Geometry: final body of the model. Coordinates: model frame, mm. Round coordinates to 2 decimals unless told otherwise and drop trailing zeros. Loops run counter-clockwise (first coordinate to the right, second up) from the corner with the lowest first, then second, coordinate; pieces in that order, holes last. Notation, with made-up numbers: M 39,19 L 91,19 A27 cw 91,44 Z; hole C -14,49 d9. An arc over 180 degrees is marked long. Answer as a JSON object with one key per item and string values.
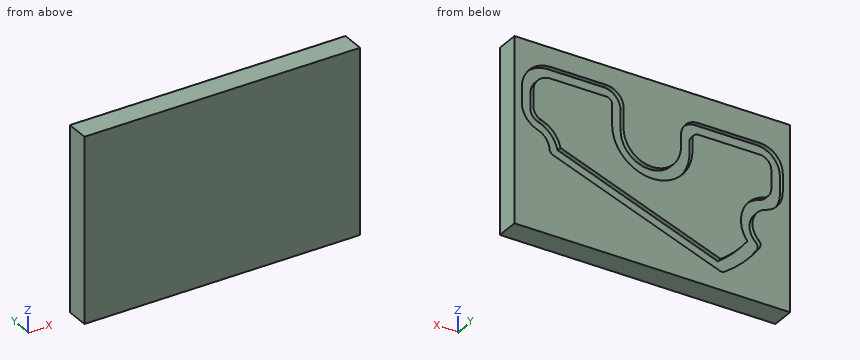
```python
from build123d import *

# Parameters (mm, degrees)
BOSS_EXTRUDE1_DEPTH = 2.54
BOSS_EXTRUDE2_DEPTH = 10.16
BOSS_EXTRUDE4_DEPTH = 2.54
FILLET1_R           = 3.175
FILLET2_R           = 3.175
FILLET3_R           = 3.175


with BuildPart() as part:
    # Sketch1 → Boss-Extrude1 (new body)
    with BuildSketch(Plane(origin=(0, 0, 0), x_dir=(1, 0, 0), z_dir=(0, 1, 0))):
        with BuildLine():
            Line((-59.436, -9.652), (-25.4, -9.652))
            ThreePointArc((-25.4, -9.652), (-23.15493597, -8.72206403), (-22.225, -6.477))
            Line((-22.225, -6.477), (-22.225, 0))
            ThreePointArc((-22.225, 0), (0, 22.225), (22.225, 0))
            Line((22.225, 0), (22.225, -11.049))
            ThreePointArc((22.225, -11.049), (23.15493597, -13.29406403), (25.4, -14.224))
            Line((25.4, -14.224), (56.134, -14.224))
            ThreePointArc((56.134, -14.224), (62.958994652, -11.396994652), (65.786, -4.572))
            Line((65.786, -4.572), (65.786, 3.786270628))
            ThreePointArc((65.786, 3.786270628), (64.573284533, 7.518670343), (61.398344054, 9.825451517))
            ThreePointArc((61.398344054, 9.825451517), (54.523861552, 14.288596243), (50.799961303, 21.590016478))
            Line((50.799961303, 21.590016478), (-37.803944764, 53.839200926))
            ThreePointArc((-37.803944764, 53.839200926), (-45.754351941, 47.268774836), (-52.580093852, 39.536458193))
            ThreePointArc((-52.580093852, 39.536458193), (-49.843866059, 24.02540152), (-61.180505495, 13.091032404))
            ThreePointArc((-61.180505495, 13.091032404), (-64.505522161, 10.809293437), (-65.786, 6.98536286))
            Line((-65.786, 6.98536286), (-65.786, -3.302))
            ThreePointArc((-65.786, -3.302), (-63.926128061, -7.792128061), (-59.436, -9.652))
        make_face()
    extrude(amount=BOSS_EXTRUDE1_DEPTH)

    # Sketch2 → Boss-Extrude2 (add)
    with BuildSketch(Plane.XZ):
        Polygon((-76.199999672, 30.988), (-76.199999672, -70.600237501), (76.199999874, -70.612), (76.200000328, 30.988), align=None)
    extrude(amount=BOSS_EXTRUDE2_DEPTH)

    # Sketch9 → Boss-Extrude4 (add)
    with BuildSketch(Plane(origin=(0, 2.54, 0), x_dir=(1, 0, 0), z_dir=(0, 1, 0))):
        Polygon((76.200000328, -30.988), (76.199999874, 70.612), (-76.199999672, 70.600237501), (-76.199999672, -30.988), align=None)
        with BuildLine():
            Line((15.875, 0), (15.875, -11.049))
            ThreePointArc((15.875, -11.049), (18.664807909, -17.784192091), (25.4, -20.574))
            Line((25.4, -20.574), (56.134, -20.574))
            ThreePointArc((56.134, -20.574), (67.449122713, -15.887122713), (72.136, -4.572))
            Line((72.136, -4.572), (72.136, 3.786270628))
            ThreePointArc((72.136, 3.786270628), (69.710569066, 11.251070057), (63.360688108, 15.864632407))
            ThreePointArc((63.360688108, 15.864632407), (58.26569903, 19.828002779), (56.883535343, 26.133305464))
            Line((56.883535343, 26.133305464), (-38.653299329, 60.905869561))
            ThreePointArc((-38.653299329, 60.905869561), (-51.084372013, 50.931222566), (-61.021650194, 38.47025739))
            ThreePointArc((-61.021650194, 38.47025739), (-55.422413128, 28.186543533), (-62.925010989, 19.196701948))
            ThreePointArc((-62.925010989, 19.196701948), (-69.575044323, 14.633224013), (-72.136, 6.98536286))
            Line((-72.136, 6.98536286), (-72.136, -3.302))
            ThreePointArc((-72.136, -3.302), (-68.416256121, -12.282256121), (-59.436, -16.002))
            Line((-59.436, -16.002), (-25.4, -16.002))
            ThreePointArc((-25.4, -16.002), (-18.664807909, -13.212192091), (-15.875, -6.477))
            Line((-15.875, -6.477), (-15.875, 0))
            ThreePointArc((-15.875, 0), (0, 15.875), (15.875, 0))
        make_face(mode=Mode.SUBTRACT)
    extrude(amount=-BOSS_EXTRUDE4_DEPTH)

    # Fillet1
    fillet1_edges = [part.edges().sort_by_distance(p)[0] for p in [
        (-38.653299329, 1.27, -60.905869561),
    ]]
    fillet(fillet1_edges, radius=FILLET1_R)

    # Fillet2
    fillet2_edges = [part.edges().sort_by_distance(p)[0] for p in [
        (56.883535343, 1.27, -26.133305464),
    ]]
    fillet(fillet2_edges, radius=FILLET2_R)

    # Fillet3
    fillet3_edges = [part.edges().sort_by_distance(p)[0] for p in [
        (-61.021650194, 1.27, -38.47025739),
    ]]
    fillet(fillet3_edges, radius=FILLET3_R)


solid = part.part
```
1) Cut plane B-B on z = -31. Return the cut outline in (x, y), and give its area (3 significant figures).
Geometry results:
{"outline": "M -76.2,-10.16 L 76.2,-10.16 L 76.2,2.54 L 43.51,2.54 L 43.51,0 L 24.95,0 L 24.95,2.54 L -49.12,2.54 L -49.12,0 L -55.53,0 L -55.53,2.54 L -76.2,2.54 Z", "area": "1,870 mm2"}
2) First-contact query: pin 1 (6 mm diameter, centred on x = -19.5, y = -4.5, fed in from -Z). Flat tip, straight axial feed; report the tip coordinate or a pass-through.
Geometry results:
{"pin 1": "z = -70.6"}
3) Cut plane C-C on z = -11.5. Return the cut outline in (x, y), and give its area (3 significant figures).
Geometry results:
{"outline": "M -76.2,-10.16 L 76.2,-10.16 L 76.2,2.54 L 69.53,2.54 L 69.53,0 L 57.83,0 L 57.83,2.54 L 19.02,2.54 L 19.02,0 L 10.94,0 L 10.94,2.54 L -10.94,2.54 L -10.94,0 L -19.02,0 L -19.02,2.54 L -63.9,2.54 L -63.9,0 L -71.31,0 L -71.31,2.54 L -76.2,2.54 Z", "area": "1,850 mm2"}
4) Cut plane A-A on x = -4. Return the cut outline in (y, z), and give its area (3 significant figures).
Geometry results:
{"outline": "M -10.16,-70.61 L 2.54,-70.61 L 2.54,-48.29 L 0,-48.29 L 0,-41.54 L 2.54,-41.54 L 2.54,-21.86 L 0,-21.86 L 0,-15.36 L 2.54,-15.36 L 2.54,30.99 L -10.16,30.99 Z", "area": "1,260 mm2"}
5) Line query: probe 1 along Z at (x, y) = (-6, 2); probe 2 along Z at (x, y) = (28.5, -2.75); probe 3 along X at (y, z) = (1.5, -20.5). Output: solid intervals per line, ascending.
Geometry results:
{"probe 1": "-70.61 to -49.02, -42.26 to -21.4, -14.7 to 30.99", "probe 2": "-70.61 to 30.99", "probe 3": "-76.2 to -60.08, -51.46 to -8.58, 8.58 to 51.07, 57.88 to 76.2"}
